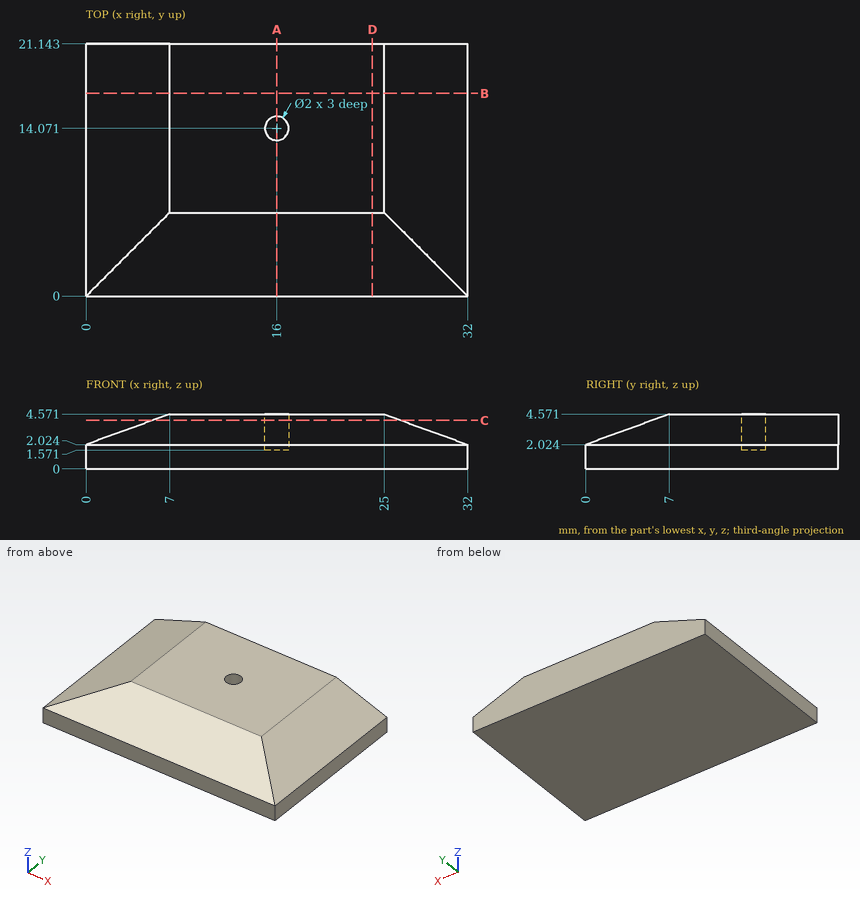
Print and shaded views of the part. All mm, measured from the part's lowest x, y and z. Coordinates: 2 decimals unless noted, no trailing zeros. Write each loop counter-clockwise with the first axis right and the second up, starting at its lowest first coordinate (ties: lowest second). Pieces come first, ordered by that corner, then holes. Notation, with made-up numbers: (0.5, 25) - (8.5, 25) arc R21 cw to (8.5, 58) - close; hole circle Ø7 at (45, -30.5). An arc over 180 degrees is marked (long way). One line per question, with ' | ' between items. Start each with the question number.
Q1. Cut at B-B, the plane y = 17. List the corners of the cut face in (x, z).
Q2. Cut at C-C, the plane z = 4.05. List the corners of the cut face in (x, y), then the cut area to 3 significant figures.
Q3. Drill centre lines: line 1 (Y direction, x = 16, z = 1.8); line 2 (Z direction, x = 5, y = 11); line 3 (Z direction, x = 4.5, y = 1). Where is each one in solid material? Low to high. Write a range as [from, to].
Q4. Cut at A-A, the plane x = 16. List the corners of the cut face in (y, z).
Q5. Cut at D-D, the plane x = 24. List the corners of the cut face in (y, z).
Q6. Pin check, flat tip, straight feed: pin 1 (2 mm diameter, centred on x = 16.5, y = 14.5, fed in from +Z). Stop position of the tip, or through.
Answer below:
1) outline: (0, 0) - (32, 0) - (32, 2.02) - (25, 4.57) - (7, 4.57) - (0, 2.02) - close
2) outline: (5.57, 5.57) - (26.43, 5.57) - (26.43, 21.14) - (5.57, 21.14) - close; hole circle Ø2 at (16, 14.07) | area: 322 mm^2
3) line 1: [0, 13.07], [15.07, 21.14] | line 2: [0, 3.84] | line 3: [0, 2.39]
4) outline: (0, 0) - (21.14, 0) - (21.14, 4.57) - (15.07, 4.57) - (15.07, 1.57) - (13.07, 1.57) - (13.07, 4.57) - (7, 4.57) - (0, 2.02) - close
5) outline: (0, 0) - (21.14, 0) - (21.14, 4.57) - (7, 4.57) - (0, 2.02) - close
6) pin 1: z = 4.57
